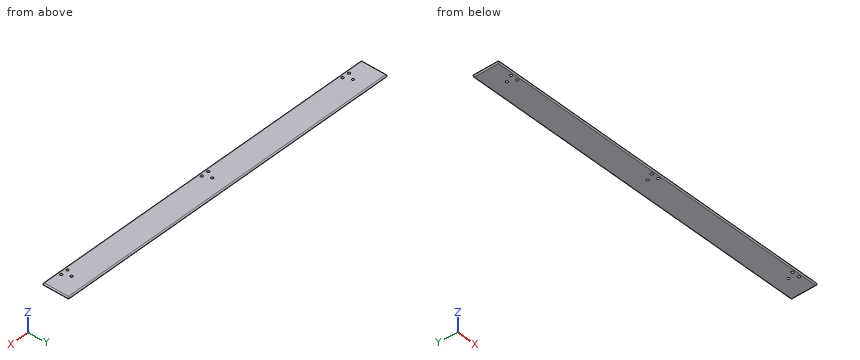
from build123d import *

# Parameters (mm, degrees)
F0_R     = 3.5
F1_DEPTH = 6
F2_R     = 2.99999


# Not quite as in the source:
# - a fillet or chamfer is up to 0.001 mm smaller than in the source, because OpenCascade refuses the exact size


with BuildPart() as f1:
    # F0 (on Top) → F1 (new body)
    with BuildSketch(Plane.XY):
        with BuildLine():
            Line((833.1764324449, 34.7622951977), (-158.1848585529, 34.7622951977))
            ThreePointArc((-158.1848585529, 34.7622951977), (-160.3061788964, 33.8836155413), (-161.1848585529, 31.7622951977))
            Line((-161.1848585529, 31.7622951977), (-161.1848585529, -35.2377048023))
            ThreePointArc((-161.1848585529, -35.2377048023), (-160.3061788964, -37.3590251459), (-158.1848585529, -38.2377048023))
            Line((-158.1848585529, -38.2377048023), (833.1764324449, -38.2377048023))
            ThreePointArc((833.1764324449, -38.2377048023), (835.2977527885, -37.3590251459), (836.1764324449, -35.2377048023))
            Line((836.1764324449, -35.2377048023), (836.1764324449, 31.7622951977))
            ThreePointArc((836.1764324449, 31.7622951977), (835.2977527885, 33.8836155413), (833.1764324449, 34.7622951977))
        make_face()
        with Locations((-111.1848585529, -28.2377048023)):
            Circle(F0_R, mode=Mode.SUBTRACT)
        with Locations((-91.1848585529, -28.2377048023)):
            Circle(F0_R, mode=Mode.SUBTRACT)
        with Locations((328.8151414471, -28.2377048023)):
            Circle(F0_R, mode=Mode.SUBTRACT)
        with Locations((-101.1848585529, -8.2377048023)):
            Circle(F0_R, mode=Mode.SUBTRACT)
        with Locations((348.8151414471, -28.2377048023)):
            Circle(F0_R, mode=Mode.SUBTRACT)
        with Locations((768.8151414471, -28.2377048023)):
            Circle(F0_R, mode=Mode.SUBTRACT)
        with Locations((788.8151414471, -28.2377048023)):
            Circle(F0_R, mode=Mode.SUBTRACT)
        with Locations((338.8151414471, -8.2377048023)):
            Circle(F0_R, mode=Mode.SUBTRACT)
        with Locations((778.8151414471, -8.2377048023)):
            Circle(F0_R, mode=Mode.SUBTRACT)
    extrude(amount=F1_DEPTH)

    # F2 (radius 3 in the source; OpenCascade refuses exactly that, so slightly less here)
    f2_edges = [f1.edges().sort_by_distance(p)[0] for p in [
        (836.176432, -35.237705, 3),
        (836.176432, 31.762295, 3),
        (836.176432, -1.737705, 0),
        (836.176432, -1.737705, 6),
    ]]
    fillet(f2_edges, radius=F2_R)


solid = f1.part
Check sheet for the modelled part. Datum: model origin and axes. Units: mm. Give positions to 0.01 mm unless a question says otherwise; leave off trailing zeros. Answer as CSV lines item,"result". Start each with the question number.
Item 1: Gauge pin test, flat end, axial feed: P1, Ø2, axis at x = 717.5, z = 1.5, coming from the +Y side. Record the tip position at first contact, or that the pin passes through.
Item 2: Cross-section at B-B on z = 4.45. State how many separate pieces and enclosed holes the cut face has, plus the area to 3 significant figures.
Item 3: Thickness scan on line 1 (X direction, y = -8, z = 2); line 2 (X direction, y = -13.5, z = 2.6); line 3 (X direction, y = 6, z = 2.4). Record the ranges inside material, lowest first. Write a range as [from, to].
Established:
1,P1,"stops at y = 34.72"
2,separate pieces,"1"
2,enclosed holes,"9"
2,area,"71,700 mm^2"
3,line 1,"x = [-161.01, -104.68], [-97.69, 335.32], [342.31, 775.32], [782.31, 836]"
3,line 2,"x = [-161.16, 836.15]"
3,line 3,"x = [-161.12, 836.12]"
